from build123d import *

# Parameters (mm, degrees)
F0_R      = 40
F0_R_2    = 35
F1_DEPTH  = 400
F3_R      = 44
F3_R_2    = 39.15
F4_DEPTH  = 2.5
F6_R      = 42.5
F6_R_2    = 39.15
F7_DEPTH  = 2.5
F10_R     = 42.5
F10_R_2   = 39.15
F11_DEPTH = 2.5
F13_R     = 42.5
F13_R_2   = 39.15
F14_DEPTH = 2.5
F16_R     = 44
F16_R_2   = 39.15
F17_DEPTH = 2.5
F19_R     = 44
F19_R_2   = 39.15
F20_DEPTH = 2.5
F22_R     = 42.5
F22_R_2   = 39.15
F23_DEPTH = 2.5
F25_R     = 44
F25_R_2   = 39.15
F26_DEPTH = 2.5
F28_R     = 44
F28_R_2   = 39.15
F29_DEPTH = 2.5


with BuildPart() as f1:
    # F0 (on Front) → F1 (new body)
    with BuildSketch(Plane.XZ):
        Circle(F0_R)
        Circle(F0_R_2, mode=Mode.SUBTRACT)
    extrude(amount=F1_DEPTH)

    # F3 (on offset) → F4 (cut)
    with BuildSketch(Plane.XZ.offset(20)):
        Circle(F3_R)
        Circle(F3_R_2, mode=Mode.SUBTRACT)
    extrude(amount=F4_DEPTH, mode=Mode.SUBTRACT)

    # F6 (on offset) → F7 (cut)
    with BuildSketch(Plane.XZ.offset(55.5)):
        Circle(F6_R)
        Circle(F6_R_2, mode=Mode.SUBTRACT)
    extrude(amount=F7_DEPTH, mode=Mode.SUBTRACT)

    # F10 (on offset) → F11 (cut)
    with BuildSketch(Plane.XZ.offset(480)):
        Circle(F10_R)
        Circle(F10_R_2, mode=Mode.SUBTRACT)
    extrude(amount=-F11_DEPTH, mode=Mode.SUBTRACT)

    # F13 (on offset) → F14 (cut)
    with BuildSketch(Plane.XZ.offset(444.5)):
        Circle(F13_R)
        Circle(F13_R_2, mode=Mode.SUBTRACT)
    extrude(amount=-F14_DEPTH, mode=Mode.SUBTRACT)

    # F16 (on offset) → F17 (cut)
    with BuildSketch(Plane.XZ.offset(590)):
        Circle(F16_R)
        Circle(F16_R_2, mode=Mode.SUBTRACT)
    extrude(amount=-F17_DEPTH, mode=Mode.SUBTRACT)

    # F19 (on offset) → F20 (cut)
    with BuildSketch(Plane.XZ.offset(600)):
        Circle(F19_R)
        Circle(F19_R_2, mode=Mode.SUBTRACT)
    extrude(amount=-F20_DEPTH, mode=Mode.SUBTRACT)

    # F22 (on offset) → F23 (cut)
    with BuildSketch(Plane.XZ.offset(294.5)):
        Circle(F22_R)
        Circle(F22_R_2, mode=Mode.SUBTRACT)
    extrude(amount=-F23_DEPTH, mode=Mode.SUBTRACT)

    # F25 (on offset) → F26 (cut)
    with BuildSketch(Plane.XZ.offset(357)):
        Circle(F25_R)
        Circle(F25_R_2, mode=Mode.SUBTRACT)
    extrude(amount=F26_DEPTH, mode=Mode.SUBTRACT)

    # F28 (on offset) → F29 (cut)
    with BuildSketch(Plane.XZ.offset(339.5)):
        Circle(F28_R)
        Circle(F28_R_2, mode=Mode.SUBTRACT)
    extrude(amount=F29_DEPTH, mode=Mode.SUBTRACT)


solid = f1.part
Read the model definition and answer for the solid it produces. Units are mm, in the model's axes. A direction names the side the tool comes from. Give positions to 0.01 mm unless a question says otherwise; leave off trailing zeros. Write each loop counter-clockwise with the first axis right and the second up, starting at its lowest first coordinate (ties: lowest second). Pieces come first, ordered by that corner, then holes. Notation, with made-up numbers: (-25.75, -9) - (8.25, -9) arc R16 ccw to (8.25, 22) - close; hole circle Ø6 at (40.5, -35.5). An arc over 180 degrees is marked (long way). Answer in a Markdown table with one row per item. Add a question column.
Item 1: Determine the mould class of faces 3 (the face through (-8.67, -38.77, -39.05)), 4 (the face through (-28, -197, -21)), 5 (the face through (26.5, -359.5, -29.4)) for opening direction Z: pulls with the +Z half, pulls with the -Z half, needs draft (parallel to the pull), parting line crosses it, or undercut.
Item 2: Section A-A, the plane y = -177 is taken. Write down the section's boundary in (x, z).
Item 3: A tool of negligible diameter and unlimited length cuts with its end or side. For faces 1 (the face through (36.165, -340.732, -14.995)), 2 (the face through (-0.2, -400, -35.4)), from which of +Z, -Z, +X, -X, +Y, -Y can it reach the whole face along a straight path? Write none if from no direction.
Item 4: Flat-ended cylindrical pins translate along their axes: P1, Ø12, axis at x = 5.5, y = -254, coming from the -Z side; P2, Ø1.5, axis at y = -117, z = 16.5, coming from the +X side; P3, Ø6, axis at x = -25, y = -335.5, coming from the +Z side. Find the tip coordinate at first contact, or state that the pin passes through.
Item 5: Find the intervals of material crossed by L1, parallel to Z at x = 0, y = -305; L2, parallel to Y at x = 20, z = -34; L3, parallel to X at y = -340, z = 20, in increasing order.
Recorded:
| question | item | result |
|---|---|---|
| 1 | face 3 | parting line crosses it |
| 1 | face 4 | undercut |
| 1 | face 5 | needs draft |
| 2 | outline | circle Ø80 at (0, 0); hole circle Ø70 at (0, 0) |
| 3 | face 1 | none |
| 3 | face 2 | +Z, -Z, +X, -X, -Y |
| 4 | P1 | stops at z = -40 |
| 4 | P2 | stops at x = 36.77 |
| 4 | P3 | stops at z = 33.41 |
| 5 | L1 | z = -40 to -35, 35 to 40 |
| 5 | L2 | y = -400 to -359.5, -357 to -342, -339.5 to -294.5, -292 to -58, -55.5 to -22.5, -20 to 0 |
| 5 | L3 | x = -33.66 to -28.72, 28.72 to 33.66 |
